```python
from build123d import *

# Parameters (mm, degrees)
EXTRUDE_1_DEPTH     = 12
SKETCH_2_R          = 9.5
SKETCH_2_R_2        = 12
CUT_EXTRUDE_1_DEPTH = 13
CUT_EXTRUDE_2_DEPTH = 6
SKETCH_4_R          = 13
CUT_EXTRUDE_3_DEPTH = 13
SKETCH_7_R          = 13.75
CUT_EXTRUDE_5_DEPTH = 2
CUT_EXTRUDE_6_DEPTH = 2


with BuildPart() as part:
    # Эскиз1 → Бобышка-Вытянуть1 (new body)
    with BuildSketch(Plane(origin=(0, 0, 0), x_dir=(1, 0, 0), z_dir=(0, 1, 0))):
        with BuildLine():
            ThreePointArc((0, -15.811388301), (50, 0), (0, 15.811388301))
            ThreePointArc((0, 15.811388301), (-50, 0), (0, -15.811388301))
        make_face()
    extrude(amount=EXTRUDE_1_DEPTH)

    # Эскиз2 → Вырез-Вытянуть1 (cut, through all)
    with BuildSketch(Plane(origin=(0, 0, 0), x_dir=(1, 0, 0), z_dir=(0, 1, 0))):
        with Locations((0, 24.25)):
            Circle(SKETCH_2_R)
        with Locations((0, -26.75)):
            Circle(SKETCH_2_R_2)
    extrude(amount=CUT_EXTRUDE_1_DEPTH, mode=Mode.SUBTRACT)

    # Эскиз3 → Вырез-Вытянуть2 (cut)
    with BuildSketch(Plane(origin=(0, 12, 0), x_dir=(1, 0, 0), z_dir=(0, 1, 0))):
        with BuildLine():
            Line((-6, 0), (-6, 3.75))
            ThreePointArc((-6, 3.75), (0, 9.75), (6, 3.75))
            Line((6, 3.75), (6, 0))
            ThreePointArc((6, 0), (30.366066361, -14.504309704), (31.5, 13.829316686))
            Line((31.5, 13.829316686), (31.5, 40))
            Line((31.5, 40), (71.5, 40))
            Line((71.5, 40), (71.5, -30))
            Line((71.5, -30), (-71.5, -30))
            Line((-71.5, -30), (-71.5, 40))
            Line((-71.5, 40), (-31.5, 40))
            Line((-31.5, 40), (-31.5, 13.829316686))
            ThreePointArc((-31.5, 13.829316686), (-30.366066361, -14.504309704), (-6, 0))
        make_face()
    extrude(amount=-CUT_EXTRUDE_2_DEPTH, mode=Mode.SUBTRACT)

    # Эскиз4 → Вырез-Вытянуть3 (cut, through all)
    with BuildSketch(Plane(origin=(0, 0, 0), x_dir=(1, 0, 0), z_dir=(0, 1, 0))):
        with Locations((-22.5, 0)):
            Circle(SKETCH_4_R)
        with Locations((22.5, 0)):
            Circle(SKETCH_4_R)
    extrude(amount=CUT_EXTRUDE_3_DEPTH, mode=Mode.SUBTRACT)

    # Эскиз7 → Вырез-Вытянуть5 (cut)
    with BuildSketch(Plane.XZ):
        with Locations((-22.5, 0)):
            Circle(SKETCH_7_R)
        with Locations((22.5, 0)):
            Circle(SKETCH_7_R)
    extrude(amount=-CUT_EXTRUDE_5_DEPTH, mode=Mode.SUBTRACT)

    # Эскиз8 → Вырез-Вытянуть6 (cut)
    with BuildSketch(Plane(origin=(0, 12, 0), x_dir=(1, 0, 0), z_dir=(0, 1, 0))):
        Polygon((-9.242640687, 24.242640687), (-26.920310217, 6.564971157), (-22.67766953, 2.32233047), (-5, 20), align=None)
        Polygon((9.242640687, 24.242640687), (26.920310217, 6.564971157), (22.67766953, 2.32233047), (5, 20), align=None)
    extrude(amount=-CUT_EXTRUDE_6_DEPTH, mode=Mode.SUBTRACT)


solid = part.part
```
CAD build for the part. Positions are in the model's coordinates, mm. A direction names the side the tool comes from. Round coordinates to 2 decimals unless told otherwise and drop trailing zeros. Order: outer loops, then holes, each group sorted by start corner. A loop starts at its lowest first (then second) coordinate and runs counter-clockwise, first axis right, second up. Notation, with made-up numbers: (42.5, 63.25) - (58.5, 63.25) arc R15 ccw to (58.5, 67.25) - close; hole circle Ø10 at (-26, 13). An arc over 180 degrees is marked (long way). Answer in a Markdown table with one row per item. Add a question column.
(1) 3-axis set-ups, long thin cutter, end or side, ignore diameter. For faces 4 (the face through (1, 6, 6)), 5 (the face through (-0.13, 9.04, -9.75)), 6 (the face through (-36.237, 0.986, 0.605)), 7 (the face through (-46.302, 4.583, -13.774)): which of +Z, -Z, +X, -X, +Y, -Y reach the whole face in a straight line?
(2) Band-saw the part on A-A on y = 8.25. List the corners of the cut face in (x, z).
(3) Band-saw the part on B-B on x = 22.5. List the corners of the cut face in (y, z), and give its area (3 significant figures).
(4) Band-saw the part on C-C on z = 22. List the corners of the cut face in (x, y).
(5) Mould opens along X. For faces 1 (the face through (31.5, 9, -20)), 2 (the face through (14.981, 11.014, -18.504)), 3 (the face through (-31.5, 9, -20)) say: +X half, -X half, draft (parallel to the pull), parting line (faces both ways), or undercut.
(6) Band-saw the part on D-D on z = -21.5. List the corners of the cut face in (x, y), and give its area (3 significant figures).
(7) Drop flat-ended pins along their axis: pin 1 Ø1.9 at (y, z) = (9, -2.5) entering from +X; pin 2 Ø5 at (y, z) = (9, -21.5) entering from +X; pin 3 Ø4 at (y, z) = (6, 20.5) entering from +X. Give the stop position or say it passes through.
(8) Probe L1, parallel to X at y = 4.75, z = 0; L2, parallel to Z at x = -22.5, y = 9.75; L3, parallel to X at y = 2.5, z = 9. List the from-to ranges inside material, lowest first. Write a range as [from, to].
Data:
| question | item | result |
|---|---|---|
| 1 | face 4 | +Y |
| 1 | face 5 | +Z, +Y |
| 1 | face 6 | -Y |
| 1 | face 7 | +Y, -Y |
| 2 | outline | (-31.5, -25.99) arc R27.5 ccw to (-9.5, -24.23) arc R9.5 cw to (9.5, -24.23) arc R27.5 ccw to (31.5, -25.99) - (31.5, -13.83) arc R16.5 ccw (long way) to (6, 0) - (6, -3.75) arc R6 cw to (-6, -3.75) - (-6, 0) arc R16.5 ccw (long way) to (-31.5, -13.83) - close; hole circle Ø26 at (-22.5, 0); hole circle Ø26 at (22.5, 0) |
| 3 | outline | (0, -27.5) - (12, -27.5) - (12, -13) - (2, -13) - (2, -13.75) - (0, -13.75) - close; (0, 13.75) - (2, 13.75) - (2, 13) - (12, 13) - (12, 16.5) - (6, 16.5) - (6, 27.5) - (0, 27.5) - close |
| 3 | area | 279 mm^2 |
| 4 | outline | (-39, 0) - (-11.02, 0) - (-11.02, 6) - (-39, 6) - close; (11.02, 0) - (39, 0) - (39, 6) - (11.02, 6) - close |
| 5 | face 1 | +X half |
| 5 | face 2 | undercut |
| 5 | face 3 | -X half |
| 6 | outline | (-39.65, 0) - (-9.09, 0) - (-9.09, 10) - (-11.99, 10) - (-11.99, 12) - (-31.5, 12) - (-31.5, 6) - (-39.65, 6) - close; (9.09, 0) - (39.65, 0) - (39.65, 6) - (31.5, 6) - (31.5, 12) - (11.99, 12) - (11.99, 10) - (9.09, 10) - close |
| 6 | area | 624 mm^2 |
| 7 | pin 1 | stops at x = 38.93 |
| 7 | pin 2 | stops at x = 31.5 |
| 7 | pin 3 | stops at x = 42.85 |
| 8 | L1 | x = [-50, -35.5], [-9.5, 9.5], [35.5, 50] |
| 8 | L2 | z = [-27.5, -13], [13, 16.5] |
| 8 | L3 | x = [-48.49, -31.88], [-13.12, 13.12], [31.88, 48.49] |
